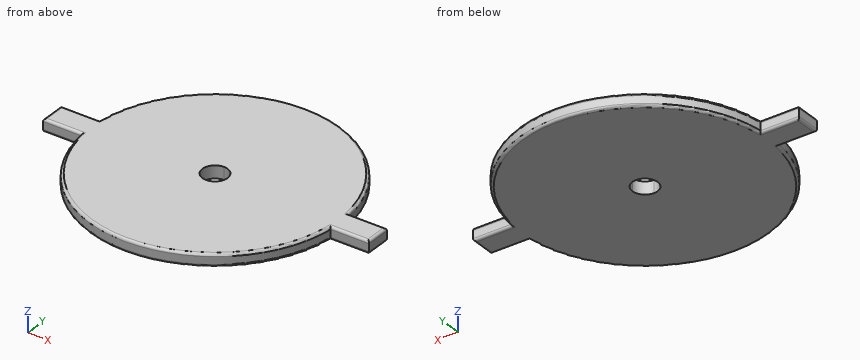
from build123d import *

# Parameters (mm, degrees)
F3_DEPTH = 1.27
F1_R     = 0.254
F2_R     = 0.254


with BuildPart() as f3:
    # F0 (on Top) → F3 (new body)
    with BuildSketch(Plane.XY):
        with BuildLine():
            ThreePointArc((-12.6363404513, -1.27), (0, -12.7), (12.6363404513, -1.27))
            Line((12.6363404513, -1.27), (0, -1.27))
            Line((0, -1.27), (-12.6363404513, -1.27))
        make_face()
        with BuildLine():
            Line((6.5e-09, 1.27), (12.6363404513, 1.27))
            ThreePointArc((12.6363404513, 1.27), (0, 12.7), (-12.6363404513, 1.27))
            Line((-12.6363404513, 1.27), (6.5e-09, 1.27))
        make_face()
        with BuildLine():
            ThreePointArc((12.6363404513, 1.27), (12.6840751285, 0.6357972433), (12.7, 0))
            ThreePointArc((12.7, 0), (12.6840751285, -0.6357972433), (12.6363404513, -1.27))
            Line((12.6363404513, -1.27), (16.51, -1.27))
            Line((16.51, -1.27), (16.51, 1.27))
            Line((16.51, 1.27), (12.6363404513, 1.27))
        make_face()
        with BuildLine():
            Line((6.5e-09, 1.27), (-12.6363404513, 1.27))
            ThreePointArc((-12.6363404513, 1.27), (-12.7, 0), (-12.6363404513, -1.27))
            Line((-12.6363404513, -1.27), (0, -1.27))
            ThreePointArc((0, -1.27), (-1.27, 3.2e-09), (6.5e-09, 1.27))
        make_face()
        with BuildLine():
            ThreePointArc((-12.6363404513, -1.27), (-12.7, 0), (-12.6363404513, 1.27))
            Line((-12.6363404513, 1.27), (-16.51, 1.27))
            Line((-16.51, 1.27), (-16.51, -1.27))
            Line((-16.51, -1.27), (-12.6363404513, -1.27))
        make_face()
        with BuildLine():
            ThreePointArc((12.6363404513, -1.27), (12.6840751285, -0.6357972433), (12.7, 0))
            ThreePointArc((12.7, 0), (12.6840751285, 0.6357972433), (12.6363404513, 1.27))
            Line((12.6363404513, 1.27), (6.5e-09, 1.27))
            ThreePointArc((6.5e-09, 1.27), (0.8980256144, 0.8980256098), (1.27, 0))
            ThreePointArc((1.27, 0), (0.8980256121, -0.8980256121), (0, -1.27))
            Line((0, -1.27), (12.6363404513, -1.27))
        make_face()
    extrude(amount=F3_DEPTH)

    # F1
    f1_edges = [f3.edges().sort_by_distance(p)[0] for p in [
        (0, 12.7, 1.27),
        (-14.57317, 1.27, 1.27),
        (-14.57317, -1.27, 1.27),
        (0, -12.7, 1.27),
        (-16.51, 0, 1.27),
        (14.57317, 1.27, 1.27),
        (14.57317, -1.27, 1.27),
        (16.51, 0, 1.27),
    ]]
    fillet(f1_edges, radius=F1_R)

    # F2
    f2_edges = [f3.edges().sort_by_distance(p)[0] for p in [
        (14.57317, -1.27, 0),
        (16.51, 0, 0),
        (14.57317, 1.27, 0),
        (0, 12.7, 0),
        (-14.57317, 1.27, 0),
        (-14.57317, -1.27, 0),
        (0, -12.7, 0),
        (-16.51, 0, 0),
    ]]
    fillet(f2_edges, radius=F2_R)


solid = f3.part
Geometry: final body of the model. Coordinates: model frame, mm. Give positions to 0.01 mm unless a question says otherwise; leave off trailing zeros. Loops run counter-clockwise (first coordinate to the right, second up) from the corner with the lowest first, then second, coordinate; pieces in that order, holes last. Notation, with made-up numbers: (-36, 68) - (16, 68) arc R28 cw to (16, 86) - close; hole circle Ø5 at (75, 60). An arc over 180 degrees is marked (long way). One line per question, with ' | ' between items. Start each with the question number.
(1) Ray query, line 1 (Y direction, x = 0.5, z = 0.3); line 2 (X direction, y = 0.25, z = 1.15); line 3 (Y direction, x = -1, z = 0.3). Return the intervals inside material, ascending. Write a range as from..to.
(2) Section query B-B on x = -13.5. Return loops of the section in (y, z), then the cut area to 3 significant figures.
(3) Section query A-A on z = 0.6. Return loops of the section in (x, y), then the cut area to 3 significant figures.
The answers:
1) line 1: -12.69..-1.17, 1.17..12.69 | line 2: -16.47..-1.25, 1.25..16.47 | line 3: -12.66..-0.78, 0.78..12.66
2) outline: (-1.27, 0.25) arc R0.25 ccw to (-1.02, 0) - (1.02, 0) arc R0.25 ccw to (1.27, 0.25) - (1.27, 1.02) arc R0.25 ccw to (1.02, 1.27) - (-1.02, 1.27) arc R0.25 ccw to (-1.27, 1.02) - close | area: 3.17 mm2
3) outline: (-16.51, -1.27) - (-12.64, -1.27) arc R12.7 ccw to (12.64, -1.27) - (16.51, -1.27) - (16.51, 1.27) - (12.64, 1.27) arc R12.7 ccw to (-12.64, 1.27) - (-16.51, 1.27) - close; hole circle Ø2.54 at (0, 0) | area: 521 mm2
